```python
from build123d import *

# Parameters (mm, degrees)
BOSS_EXTRUDE1_DEPTH = 170
SKETCH2_W           = 154
SKETCH2_H           = 50
CUT_EXTRUDE1_DEPTH  = 10
CUT_EXTRUDE2_DEPTH  = 160
SKETCH4_W           = 51
SKETCH4_H           = 20
SKETCH4_W_2         = 72
SKETCH4_H_2         = 27
CUT_EXTRUDE3_DEPTH  = 10


with BuildPart() as part:
    # Sketch1 → Boss-Extrude1 (new body)
    with BuildSketch(Plane(origin=(0, 0, 0), x_dir=(0, 0, -1), z_dir=(1, 0, 0))):
        Polygon((-54.32397065, 28.139382559), (15.67602935, 28.139382559), (15.67602935, -31.860617441), (-104.32397065, -31.860617441), (-104.32397065, -21.860617441), align=None)
    extrude(amount=BOSS_EXTRUDE1_DEPTH)

    # Sketch2 → Cut-Extrude1 (cut)
    with BuildSketch(Plane(origin=(0, 28.139382559, 0), x_dir=(1, 0, 0), z_dir=(0, 1, 0))):
        with Locations((85, -19.32397065)):
            Rectangle(SKETCH2_W, SKETCH2_H)
    extrude(amount=-CUT_EXTRUDE1_DEPTH, mode=Mode.SUBTRACT)

    # Sketch3 → Cut-Extrude2 (cut)
    with BuildSketch(Plane(origin=(170, 0, 0), x_dir=(0, 0, -1), z_dir=(1, 0, 0))):
        Polygon((-51.40243063, 23.139382559), (10.67602935, 23.139382559), (10.67602935, -26.860617441), (-99.32397065, -26.860617441), (-99.32397065, -24.782157461), align=None)
    extrude(amount=-CUT_EXTRUDE2_DEPTH, mode=Mode.SUBTRACT)

    # Sketch4 → Cut-Extrude3 (cut)
    with BuildSketch(Plane(origin=(0, 41.231676605, 41.231676605), x_dir=(1, 0, 0), z_dir=(0, 0.7071067811865474, 0.7071067811865477))):
        with Locations((41.5, -36.515299802)):
            Rectangle(SKETCH4_W, SKETCH4_H)
        with Locations((128.5, -36.515299802)):
            Rectangle(SKETCH4_W, SKETCH4_H)
        with Locations((85, -67.72597792)):
            Rectangle(SKETCH4_W_2, SKETCH4_H_2)
    extrude(amount=-CUT_EXTRUDE3_DEPTH, mode=Mode.SUBTRACT)


solid = part.part
```
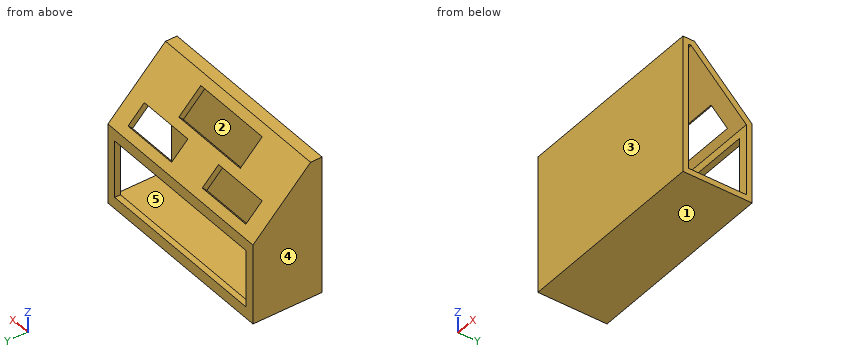
The listing builds one solid part. Answer for the finished solid, in the listing's coordinates (mm). Face numbers are marked on the shaded views. A direction names the side the tool comes from. Round coordinates to 2 decimals unless told otherwise and drop trailing zeros. Order: outer loops, then holes, each group sorted by start corner. A loop starts at its lowest first (then second) coordinate and runs counter-clockwise, first axis right, second up. Notation, with made-up numbers: (83, 30) - (120, 30) arc R22 cw to (120, 43) - close; hole circle Ø11 at (60, 30.5). An arc over 180 degrees is marked (long way). Put each result on its own line as item: value. Start each with the question number.
(1) For the marked faces 4 and 5, determine the directions among +Z, -Z, +X, -X, +Y, -Y from which every point of the face is accessible in a straight line to the end or side of a thin tool.
(2) Find section D-D (y = 15.5). Give the vertices of the cut face in (x, z), plus the area to 3 significant figures.
(3) Given P1, Ø2, axis at x = 61.5, z = 20, coming from the +Y side; P2, Ø1, axis at x = 54.5, y = 6, coming from the +Z side; P3, Ø1, axis at x = 98, z = 80, coming from the +Y side, each flat-ended and moving along its own axis, determine where each tip first touches the part or whether it passes through.
(4) Determine the mould class of the marked faces 1, 2 and 3 for opening direction Y: released by +Y, released by -Y, zero draft, split by the parting line, or undercut.
(5) Find section C-C (x = 149.5). Give the vertices of the cut face in (y, z).
(6) Find section A-A (x = 111). Give the vertices of the cut face in (y, z).
(7) Straight lines are drawn through the part: probe 1 along X at (y, z) = (25.5, 15.5); probe 2 along Y at (x, z) = (135, -6); probe 3 along Z at (x, y) = (49, 17.5). For each, find the intervals that lie inside material, in ascending order. Write a range as from..to.
(8) Find section B-B (z = 41). Give the vertices of the cut face in (x, y).
Reply:
1. face 4: +Z, -Z, -X, +Y, -Y
1. face 5: +X
2. outline: (0, -15.68) - (170, -15.68) - (170, -10.68) - (10, -10.68) - (10, 59.04) - (16, 59.04) - (16, 66.96) - (0, 66.96) - close; (67, 59.04) - (103, 59.04) - (103, 66.96) - (67, 66.96) - close; (154, 59.04) - (170, 59.04) - (170, 66.96) - (154, 66.96) - close
2. area: 2,090 mm^2
3. P1: y = -26.86
3. P2: z = 76.96
3. P3: y = 2.96
4. face 1: zero draft
4. face 2: undercut
4. face 3: released by -Y
5. outline: (-31.86, -15.68) - (28.14, -15.68) - (28.14, -5.68) - (23.14, -5.68) - (23.14, -10.68) - (-26.86, -10.68) - (-26.86, 99.32) - (-24.78, 99.32) - (4.38, 70.16) - (8.34, 74.12) - (-21.86, 104.32) - (-31.86, 104.32) - close; (18.52, 56.02) - (23.14, 51.4) - (23.14, 44.32) - (28.14, 44.32) - (28.14, 54.32) - (22.48, 59.98) - close
6. outline: (-31.86, -15.68) - (28.14, -15.68) - (28.14, -5.68) - (23.14, -5.68) - (23.14, -10.68) - (-26.86, -10.68) - (-26.86, 99.32) - (-24.78, 99.32) - (-20.16, 94.71) - (-16.2, 98.67) - (-21.86, 104.32) - (-31.86, 104.32) - close; (-1.07, 75.61) - (4.38, 70.16) - (8.34, 74.12) - (2.89, 79.58) - close; (18.52, 56.02) - (23.14, 51.4) - (23.14, 44.32) - (28.14, 44.32) - (28.14, 54.32) - (22.48, 59.98) - close
7. probe 1: 0..8, 162..170
7. probe 2: -31.86..-26.86, 23.14..28.14
7. probe 3: -15.68..-10.68
8. outline: (0, -31.86) - (170, -31.86) - (170, -26.86) - (10, -26.86) - (10, 18.14) - (8, 18.14) - (8, 28.14) - (0, 28.14) - close; (162, 23.14) - (170, 23.14) - (170, 28.14) - (162, 28.14) - close
